Source: three-view drawing plus pictorial views. Frame: mm from the lowest corner of the part. Give positions to 0.01 mm unless a question says otherwise; leave off trailing zeros. Order: outer loops, then holes, each group sorted by start corner. A loop starts at its lowest first (then second) coordinate and runs counter-clockwise, first axis right, second up. Notation, with made-up numbers: (75, 88) - (122, 88) arc R9 cw to (122, 95) - close; hole circle Ø3 at (-15.75, 81). An arc over 180 degrees is marked (long way). Answer in a Markdown table with one row per item. Add a question column.
1. Section query B-B on y = 25.4. Return loops of the section in (x, z) (1 decimal), and give its area (3 significant figures).
2. Ray query, line 1 (Y direction, x = 8.5, z = 25.4); line 2 (Z direction, x = 17.75, y = 24) (1 decimal); line 3 (Z direction, x = 15.25, y = 19) (1 decimal). Return the intervals inside material, ascending. Write a range as [from, to].
3. Section query A-A on z = 25.4. Return loops of the section in (x, y), and give its area (3 significant figures).
4. Section query C-C on x = 6.25. Return loops of the section in (y, z) (1 decimal).
5. Section query D-D on z = 227.5. Return loops of the section in (x, y).
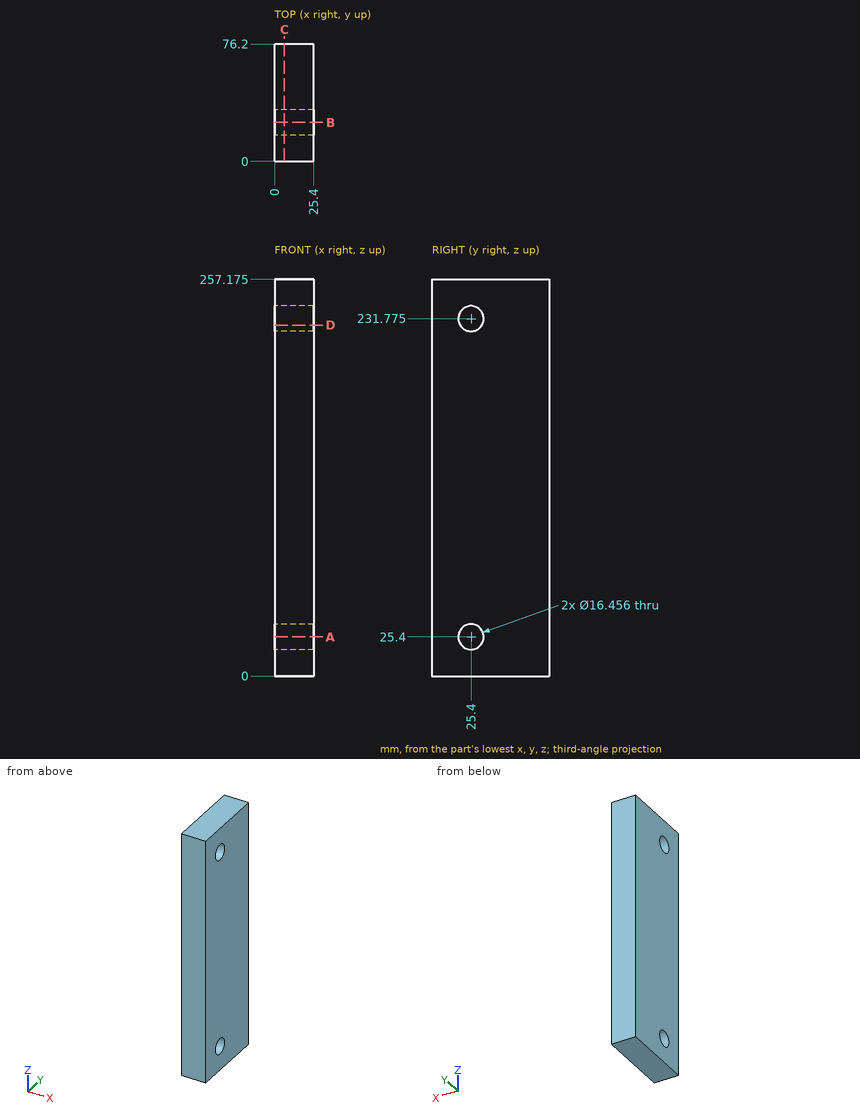
Answer:
| question | item | result |
|---|---|---|
| 1 | outline | (0, 0) - (25.4, 0) - (25.4, 17.2) - (0, 17.2) - close; (0, 33.6) - (25.4, 33.6) - (25.4, 223.5) - (0, 223.5) - close; (0, 240) - (25.4, 240) - (25.4, 257.2) - (0, 257.2) - close |
| 1 | area | 5,700 mm² |
| 2 | line 1 | y = [0, 17.17], [33.63, 76.2] |
| 2 | line 2 | z = [0, 17.3], [33.5, 223.7], [239.9, 257.2] |
| 2 | line 3 | z = [0, 20.2], [30.6, 226.6], [236.9, 257.2] |
| 3 | outline | (0, 0) - (25.4, 0) - (25.4, 17.17) - (0, 17.17) - close; (0, 33.63) - (25.4, 33.63) - (25.4, 76.2) - (0, 76.2) - close |
| 3 | area | 1,520 mm² |
| 4 | outline | (0, 0) - (76.2, 0) - (76.2, 257.2) - (0, 257.2) - close; hole circle Ø16.5 at (25.4, 25.4); hole circle Ø16.5 at (25.4, 231.8) |
| 5 | outline | (0, 0) - (25.4, 0) - (25.4, 18.37) - (0, 18.37) - close; (0, 32.43) - (25.4, 32.43) - (25.4, 76.2) - (0, 76.2) - close |
